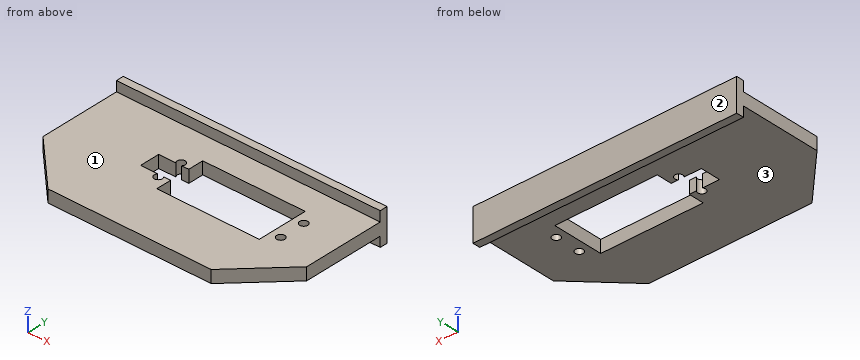
```python
from build123d import *

# Parameters (mm, degrees)
SKETCH_1_W          = 105
SKETCH_1_H          = 52.5
SKETCH_1_R          = 1.6
SKETCH_1_W_2        = 40.8
SKETCH_1_H_2        = 20.3
EXTRUDE_1_DEPTH     = 5
SKETCH_3_W          = 13
SKETCH_3_H          = 3
EXTRUDE_2_DEPTH     = 105
SKETCH_4_W          = 24
SKETCH_4_H          = 8
CUT_EXTRUDE_1_DEPTH = 118.738056719
CHAMFER_1_SIZE      = 20


with BuildPart() as part:
    # 草图1 → 凸台-拉伸1 (new body)
    with BuildSketch(Plane.XY):
        with Locations((52.5, -26.25)):
            Rectangle(SKETCH_1_W, SKETCH_1_H)
        with Locations((39.864981543, -15.671828005)):
            Circle(SKETCH_1_R, mode=Mode.SUBTRACT)
        with Locations((39.864981543, -25.821828005)):
            Circle(SKETCH_1_R, mode=Mode.SUBTRACT)
        with Locations((88.664981543, -15.671828005)):
            Circle(SKETCH_1_R, mode=Mode.SUBTRACT)
        with Locations((88.664981543, -25.821828005)):
            Circle(SKETCH_1_R, mode=Mode.SUBTRACT)
        with Locations((64.264981543, -20.746828005)):
            Rectangle(SKETCH_1_W_2, SKETCH_1_H_2, mode=Mode.SUBTRACT)
    extrude(amount=EXTRUDE_1_DEPTH)

    # 草图3 → 凸台-拉伸2 (add, through all)
    with BuildSketch(Plane.ZY):
        with Locations((2.5, 1.5)):
            Rectangle(SKETCH_3_W, SKETCH_3_H)
    extrude(amount=-EXTRUDE_2_DEPTH)

    # 草图4 → 切除-拉伸1 (cut, through all)
    with BuildSketch(Plane.XY.offset(5)):
        with Locations((43.864981543, -20.746828005)):
            Rectangle(SKETCH_4_W, SKETCH_4_H)
    extrude(amount=-CUT_EXTRUDE_1_DEPTH, mode=Mode.SUBTRACT)

    # 倒角1
    chamfer_1_edges = [part.edges().sort_by_distance(p)[0] for p in [
        (105, -52.5, 2.5),
        (0, -52.5, 2.5),
    ]]
    chamfer(chamfer_1_edges, length=CHAMFER_1_SIZE)


solid = part.part
```
Read the model definition and answer for the solid it produces. Units are mm, in the model's axes. Face numbers are marked on the shaded views. A direction names the side the tool comes from. Give positions to 0.01 mm unless a question says otherwise; leave off trailing zeros. Write each loop counter-clockwise with the first axis right and the second up, starting at its lowest first coordinate (ties: lowest second). Pieces come first, ordered by that corner, then holes. Notation, with made-up numbers: (28, 74) -> (56, 74) arc R36 cw to (56, 113) -> close; hole circle Ø3 at (75, 27.25). An arc over 180 degrees is marked (long way). Answer in a Markdown table with one row per item.
1) Section C-C on x = 14.5 is taken. Give the vertices of the cut face in (y, z), plus the area to 3 significant figures.
Results list:
| item | result |
|---|---|
| outline | (-47, 0) -> (0, 0) -> (0, -4) -> (3, -4) -> (3, 9) -> (0, 9) -> (0, 5) -> (-47, 5) -> close |
| area | 274 mm^2 |
2) Section D-D on z = 2 is taken. Give the vertices of the cut face in (x, y), plus the area to 3 significant figures.
Results list:
| item | result |
|---|---|
| outline | (0, -32.5) -> (20, -52.5) -> (85, -52.5) -> (105, -32.5) -> (105, 3) -> (0, 3) -> close; hole (31.86, -24.75) -> (38.68, -24.75) arc R1.6 ccw (long way) to (41.05, -24.75) -> (43.86, -24.75) -> (43.86, -30.9) -> (84.66, -30.9) -> (84.66, -10.6) -> (43.86, -10.6) -> (43.86, -16.75) -> (41.05, -16.75) arc R1.6 ccw (long way) to (38.68, -16.75) -> (31.86, -16.75) -> close; hole circle Ø3.2 at (88.66, -25.82); hole circle Ø3.2 at (88.66, -15.67) |
| area | 4,470 mm^2 |
3) A tool of negligible diameter and unlimited length cuts with its end or side. For the marked faces 1, 2 and 3, from which of +Z, -Z, +X, -X, +Y, -Y can it reach the whole face along a straight path? Write none if from no direction.
Results list:
| item | result |
|---|---|
| face 1 | +Z, +X, -X, -Y |
| face 2 | +Z, -Z, +X, -X, +Y |
| face 3 | -Z, +X, -X, -Y |
4) Each of these flat-tipped pins is pushed along its axis until it touches: pin 1 Ø1.2 at (x, z) = (69.5, 6.5) entering from -Y; pin 2 Ø5 at (x, y) = (32.5, -24) entering from +Z; pin 3 Ø3 at (x, y) = (84, -8) entering from -Z. Where does it stop, or does it pass through?
Results list:
| item | result |
|---|---|
| pin 1 | y = 0 |
| pin 2 | z = 5 |
| pin 3 | z = 0 |
5) Straight lines are drawn through the part: line 1 (Y direction, x = 71, z = 2); line 2 (X direction, y = -30.5, z = 0.5); line 3 (Z direction, x = 72.5, y = -40). For each, find the intervals that lie inside material, in ascending order. Write a range as [from, to].
Results list:
| item | result |
|---|---|
| line 1 | [-52.5, -30.9], [-10.6, 3] |
| line 2 | [0, 43.86], [84.66, 105] |
| line 3 | [0, 5] |
6) Section A-A on x = 77 is taken. Give the vertices of the cut face in (y, z), plus the area to 3 significant figures.
Results list:
| item | result |
|---|---|
| outline | (-52.5, 0) -> (-30.9, 0) -> (-30.9, 5) -> (-52.5, 5) -> close; (-10.6, 0) -> (0, 0) -> (0, -4) -> (3, -4) -> (3, 9) -> (0, 9) -> (0, 5) -> (-10.6, 5) -> close |
| area | 200 mm^2 |
7) Section B-B on y = -21 is taken. Give the vertices of the cut face in (x, z).
Results list:
| item | result |
|---|---|
| outline | (0, 0) -> (31.86, 0) -> (31.86, 5) -> (0, 5) -> close; (84.66, 0) -> (105, 0) -> (105, 5) -> (84.66, 5) -> close |
